```python
from build123d import *

# Parameters (mm, degrees)
F1_DEPTH = 118.11
F2_W     = 39.04492
F2_H     = 6.477
F3_DEPTH = 118.11
F4_R     = 1.778
F5_DEPTH = 25.4


with BuildPart() as f1:
    # F0 (on Right) → F1 (new body)
    with BuildSketch(Plane.YZ):
        with BuildLine():
            ThreePointArc((0, 31.75), (8.507387, 0), (0, -31.75))
            Line((0, -31.75), (5.08, -31.75))
            ThreePointArc((5.08, -31.75), (13.587387, 0), (5.08, 31.75))
            Line((5.08, 31.75), (0, 31.75))
        make_face()
    extrude(amount=F1_DEPTH)

    # F2 (on face) → F3 (join, through all)
    with BuildSketch(Plane(origin=(0, 0, 0), x_dir=(0, -1, 0), z_dir=(-1, 0, 0))):
        with Locations((-32.289425, 6.082614)):
            Rectangle(F2_W, F2_H)
    extrude(amount=-F3_DEPTH)

    # F4 (on face) → F5 (cut)
    with BuildSketch(Plane.XY.offset(9.321114)):
        with Locations((59.055, 48.001833)):
            Circle(F4_R)
        with Locations((49.6062, 48.001833)):
            Circle(F4_R)
        with Locations((40.1574, 48.001833)):
            Circle(F4_R)
        with Locations((68.5038, 48.001833)):
            Circle(F4_R)
        with Locations((77.9526, 48.001833)):
            Circle(F4_R)
        with Locations((30.7086, 48.001833)):
            Circle(F4_R)
        with Locations((87.4014, 48.001833)):
            Circle(F4_R)
    extrude(amount=-F5_DEPTH, mode=Mode.SUBTRACT)


solid = f1.part
```
CAD build for the part. Positions are in the model's coordinates, mm. A direction names the side the tool comes from. Coordinates: 2 decimals unless noted, no trailing zeros. Loops run counter-clockwise (first coordinate to the right, second up) from the corner with the lowest first, then second, coordinate; pieces in that order, holes last. Notation, with made-up numbers: (44.25, 46) - (87.25, 46) arc R22 cw to (87.25, 85) - close; hole circle Ø3 at (22.25, 43.5). An arc over 180 degrees is marked (long way). Use CSV: the item, a comma, the result in double quotes. Start each with the question number.
Q1. Cut at C-C, the plane z = -10.5. List the corners of the cut face in (x, y), then the cut area to 3 significant figures.
Q2. Cut at A-A, the plane x = 35.5. List the corners of the cut face in (y, z).
Q3. Drop flat-ended pins along their axis: P1, Ø11.5, axis at x = 43.5, y = 38.5, coming from the +Z side; P2, Ø4, axis at x = 59.06, y = 48, coming from the -Z side; P3, Ø5, axis at x = 43.5, z = 8.5, coming from the -Y side. Give the stop position or say it passes through.
Q4. Two-plate mould, pull along Y, no slides. Class faces 3 (the cylindrical face through (79.595, 47.321, 6.128)), 4 (the cylindrical face through (58.228, 8.506, 0.465)), 5 (the flat face through (58, 33, 2.844)), 6 (the cylindrical face through (47.83, 48.08, 6.13)): +Y half, -Y half, draft (parallel to the pull), parting line (faces both ways), or undercut.
Q5. Cut at B-B, the plane y = 29.5. List the corners of the cut face in (x, z), then the cut area to 3 significant figures.
Q6. Probe probe 1 along Z at (x, y) = (38.5, 14.5); probe 2 along Y at (x, z) = (49, 29); probe 3 along Y at (x, z) = (108.5, -7). List the from-to ranges inside material, lowest first. Write a range as from..to.
Q7. 3-axis set-ups, long thin cutter, end or side, ignore diameter. For faces 1 (the cylindrical face through (89.044, 47.321, 6.128)), 2 (the flat face through (58, 33, 9.321)): which of +Z, -Z, +X, -X, +Y, -Y reach the whole face in a straight line?
Here are the results:
1,outline,"(0, 7.63) - (118.11, 7.63) - (118.11, 12.71) - (0, 12.71) - close"
1,area,"600 mm2"
2,outline,"(0, -31.75) - (5.08, -31.75) arc R63.5 ccw to (13.52, 2.84) - (51.81, 2.84) - (51.81, 9.32) - (12.9, 9.32) arc R63.5 ccw to (5.08, 31.75) - (0, 31.75) arc R63.5 cw to start"
3,P1,"z = 9.32"
3,P2,"z = 2.84"
3,P3,"y = 7.55"
4,face 3,"undercut"
4,face 4,"-Y half"
4,face 5,"draft"
4,face 6,"undercut"
5,outline,"(0, 2.84) - (118.11, 2.84) - (118.11, 9.32) - (0, 9.32) - close"
5,area,"765 mm2"
6,probe 1,"2.84..9.32"
6,probe 2,"1.5..6.58"
6,probe 3,"8.12..13.2"
7,face 1,"+Z, -Z"
7,face 2,"+Z, +X, -X, +Y"
